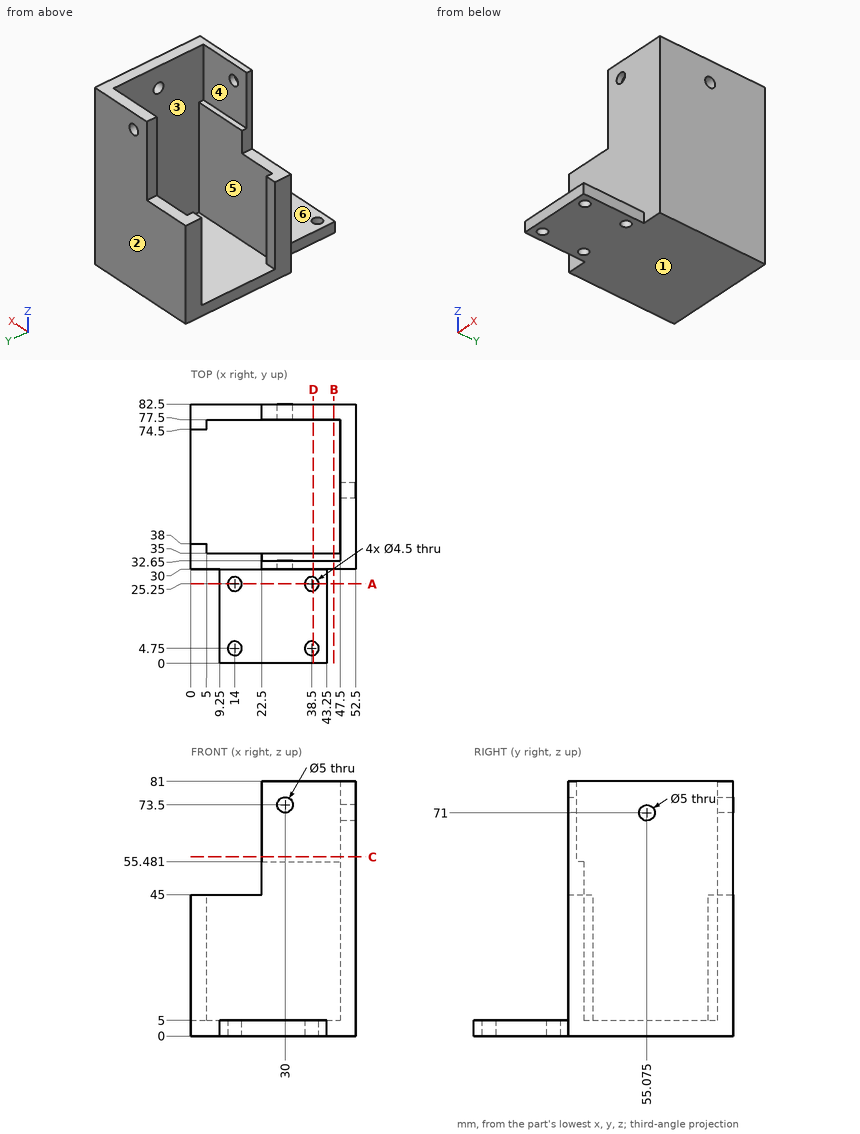
The figure shows three views and two pictorial views of one solid part (mm, origin at its lowest corner). Answer the questions. A direction names the side the tool comes from. Give positions to 0.01 mm unless a question says otherwise; leave off trailing zeros. Write each loop counter-clockwise with the first axis right and the second up, starting at its lowest first coordinate (ties: lowest second). Pieces come first, ordered by that corner, then holes. Notation, with made-up numbers: (89, 13.5) - (146, 13.5) arc R12 ccw to (146, 33.5) - close; hole circle Ø1 at (71.25, 27). An arc over 180 degrees is marked (long way). Use one line per item in the form item = value. Start each with the question number.
1) Find section B-B on x = 45.5. Determine the outline of the cut face in (y, z).
2) Flat-ended cylindrical pins translate along their axes: pin 1 Ø8 at (x, z) = (30, 73.5) entering from -Y; pin 2 Ø4 at (y, z) = (12, 2.5) entering from -X; pin 3 Ø6 at (x, y) = (14, 25.25) entering from +Z; pin 4 Ø12 at (x, y) = (21, 41) entering from -Z. Find the tip coordinate at first contact, or state that the pin passes through.
3) The mould has two halves that part along Y. Classify the marked faces 1, 2 and 3: pulls with the +Y half, pulls with the -Y half, needs draft (parallel to the pull), parting line crosses it, or undercut.
4) Consider line 1 along Y through (x, z) = (38.5, 3.2); line 2 along X through (y, z) = (25, 2); line 3 along Z through (x, y) = (30, 31.2). Determine where each line is inside the solid, lowest interval first. Write a range as from..to.
5) Find section A-A on y = 25.25. Determine the outline of the cut face in (x, z), plus the area to 3 significant figures.
6) A tool of negligible diameter and unlimited length cuts with its end or side. For the marked faces 4, 5 and 6, from which of +Z, -Z, +X, -X, +Y, -Y can it reach the whole face along a straight path? Write none if from no direction.
7) Find section C-C on z = 57. Determine the outline of the cut face in (x, y), plus the area to 3 significant figures.
8) Find section D-D on x = 39. Determine the outline of the cut face in (y, z), plus the area to 3 significant figures.
Geometry results:
q1.outline = (30, 0) - (82.5, 0) - (82.5, 81) - (77.5, 81) - (77.5, 5) - (35, 5) - (35, 55.48) - (32.65, 55.48) - (32.65, 81) - (30, 81) - close
q2.pin_1 = 30
q2.pin_2 = 9.25
q2.pin_3 = 5
q2.pin_4 = 0
q3.face_1 = needs draft
q3.face_2 = pulls with the +Y half
q3.face_3 = undercut
q4.line_1 = 0..2.5, 7..23, 27.5..82.5
q4.line_2 = 9.25..11.76, 16.24..36.26, 40.74..43.25
q4.line_3 = 0..71, 76..81
q5.outline = (9.25, 0) - (11.75, 0) - (11.75, 5) - (9.25, 5) - close; (16.25, 0) - (36.25, 0) - (36.25, 5) - (16.25, 5) - close; (40.75, 0) - (43.25, 0) - (43.25, 5) - (40.75, 5) - close
q5.area = 125 mm2
q6.face_4 = +Z, -X
q6.face_5 = +Z
q6.face_6 = +Z, +X, -X, -Y
q7.outline = (22.5, 30) - (52.5, 30) - (52.5, 82.5) - (22.5, 82.5) - (22.5, 77.5) - (47.5, 77.5) - (47.5, 32.65) - (22.5, 32.65) - close
q7.area = 454 mm2
q8.outline = (0, 0) - (2.56, 0) - (2.56, 5) - (0, 5) - close; (6.94, 0) - (23.06, 0) - (23.06, 5) - (6.94, 5) - close; (27.44, 0) - (82.5, 0) - (82.5, 81) - (77.5, 81) - (77.5, 5) - (35, 5) - (35, 55.48) - (32.65, 55.48) - (32.65, 81) - (30, 81) - (30, 5) - (27.44, 5) - close
q8.area = 1,070 mm2
